```python
from build123d import *

# Parameters (mm, degrees)
SKETCH1_W           = 50.8
SKETCH1_H           = 25.4
SKETCH1_W_2         = 47.625
SKETCH1_H_2         = 22.225
BOSS_EXTRUDE1_DEPTH = 355.6
SKETCH2_R           = 12.7
SKETCH2_R_2         = 2.54
CUT_EXTRUDE4_DEPTH  = 32.766
CUT_EXTRUDE5_REACH  = 359.41


with BuildPart() as part:
    # Sketch1 → Boss-Extrude1 (new body)
    with BuildSketch(Plane.XY):
        Rectangle(SKETCH1_W, SKETCH1_H)
        Rectangle(SKETCH1_W_2, SKETCH1_H_2, mode=Mode.SUBTRACT)
    extrude(amount=BOSS_EXTRUDE1_DEPTH)

    # Sketch2 → Cut-Extrude4 (cut)
    with BuildSketch(Plane(origin=(0, 12.7, 0), x_dir=(1, 0, 0), z_dir=(0, 1, 0))):
        with Locations(Location((0, -177.8, 0), (0, 0, 180))):
            Circle(SKETCH2_R)
        with Locations(Location((0, -152.4, 0), (0, 0, 180))):
            Circle(SKETCH2_R_2)
        with Locations(Location((0, -201.676, 0), (0, 0, 180))):
            Circle(SKETCH2_R_2)
    extrude(amount=-CUT_EXTRUDE4_DEPTH, mode=Mode.SUBTRACT)

    # Sketch3 → Cut-Extrude5 (cut, up to next)
    with BuildSketch(Plane.XZ.offset(12.7), mode=Mode.PRIVATE) as cut_extrude5_sk1:
        with BuildLine():
            ThreePointArc((-4.48e-07, 355.6), (12.899331681, 354.46174048), (25.4, 351.082140551))
            Line((25.4, 351.082140551), (25.4, 355.6))
            Line((25.4, 355.6), (-4.48e-07, 355.6))
        make_face()
    cut_extrude5_tool1 = extrude(cut_extrude5_sk1.sketch, amount=-CUT_EXTRUDE5_REACH, mode=Mode.PRIVATE) & part.part
    # Sketch3 → Cut-Extrude5 (cut, up to next)
    with BuildSketch(Plane.XZ.offset(12.7), mode=Mode.PRIVATE) as cut_extrude5_sk2:
        with BuildLine():
            Line((-25.4, 355.6), (-25.4, 351.082140551))
            ThreePointArc((-25.4, 351.082140551), (-12.899332122, 354.461740401), (-4.48e-07, 355.6))
            Line((-4.48e-07, 355.6), (-25.4, 355.6))
        make_face()
    cut_extrude5_tool2 = extrude(cut_extrude5_sk2.sketch, amount=-CUT_EXTRUDE5_REACH, mode=Mode.PRIVATE) & part.part
    # Sketch3 → Cut-Extrude5 (cut, up to next)
    with BuildSketch(Plane.XZ.offset(12.7), mode=Mode.PRIVATE) as cut_extrude5_sk3:
        with BuildLine():
            ThreePointArc((25.4, 4.436419441), (12.892263223, 1.117437052), (-2.64e-07, 0))
            Line((-2.64e-07, 0), (25.4, 0))
            Line((25.4, 0), (25.4, 4.436419441))
        make_face()
    cut_extrude5_tool3 = extrude(cut_extrude5_sk3.sketch, amount=-CUT_EXTRUDE5_REACH, mode=Mode.PRIVATE) & part.part
    # Sketch3 → Cut-Extrude5 (cut, up to next)
    with BuildSketch(Plane.XZ.offset(12.7), mode=Mode.PRIVATE) as cut_extrude5_sk4:
        with BuildLine():
            Line((-25.4, 4.436419441), (-25.4, 0))
            Line((-25.4, 0), (-2.64e-07, 0))
            ThreePointArc((-2.64e-07, 0), (-12.892263483, 1.117437097), (-25.4, 4.436419441))
        make_face()
    cut_extrude5_tool4 = extrude(cut_extrude5_sk4.sketch, amount=-CUT_EXTRUDE5_REACH, mode=Mode.PRIVATE) & part.part
    add(cut_extrude5_tool1.solids().sort_by_distance((19.0896, -12.7, 354.252078))[0], mode=Mode.SUBTRACT)
    add(cut_extrude5_tool2.solids().sort_by_distance((-19.0896, -12.7, 354.252078))[0], mode=Mode.SUBTRACT)
    add(cut_extrude5_tool3.solids().sort_by_distance((19.088205, -12.7, 1.323888))[0], mode=Mode.SUBTRACT)
    add(cut_extrude5_tool4.solids().sort_by_distance((-19.088205, -12.7, 1.323888))[0], mode=Mode.SUBTRACT)


solid = part.part
```
For this review, take the finished solid that the model builds, in its own axes (mm). A direction names the side the tool comes from. Coordinates: 2 decimals unless noted, no trailing zeros. Order: outer loops, then holes, each group sorted by start corner. A loop starts at its lowest first (then second) coordinate and runs counter-clockwise, first axis right, second up. Notation, with made-up numbers: (37, -12.5) - (64, -12.5) arc R31 cw to (64, 25.5) - close; hole circle Ø3 at (14, 50). An arc over 180 degrees is marked (long way). Answer as a JSON object with one key per item and string values. Group by question number.
1. Clearance check with flat-ended pins moving along their axes: P1, Ø20.5, axis at x = 0, z = 177.8, coming from the -Y side (1 decimal); P2, Ø8, axis at x = -7.5, y = -8, coming from the -Z side; P3, Ø6, axis at x = 0, z = 152.4, coming from the +Y side. State where each tip first meets the part, or that it passes through.
2. We need section B-B on y = -5.75. State the section outline as (x, z) points.
3. For probe 1 along Z at (x, y) = (0, -11.75); probe 2 along Y at (x, z) = (9, 106); probe 3 along X at (y, z) = (12.35, 152.4), list the stretches that pass through material, from the lowest coordinate up.
4. The part is to be moulded in two halves that separate along X. For faces 3 (the flat face through (17, -12.7, 175)), 4 (the flat face through (-16, -11.112, 175)), 5 (the flat face through (-25.4, 0, 175)), 6 (the flat face through (25.4, 0, 175)), say which applies: pulls with the +X half, pulls with the -X half, needs draft (parallel to the pull), parting line crosses it, or undercut.
5. We need section A-A on z = 138. State the section outline as (x, y) points.
6. We need section C-C on z = 177.8. State the section outline as (x, y) points.
7. For faces 1 (the flat face through (-23.812, 0, 175)), 2 (the flat face through (17, 12.7, 175)), list the 3-axis set-ups (+Z, -Z, +X, -X, +Y, -Y) from which the entire face can be reached by the end or side of a thin tool; tool diameter is ignored.
Final values:
{
 "1": {"P1": "through", "P2": "z = 0.17", "P3": "y = 12.7"},
 "2": {"outline": "(-25.4, 4.44) arc R74.93 ccw to (-23.81, 3.88) - (-23.81, 351.64) arc R73.66 ccw to (-25.4, 351.08) - close; (23.81, 3.88) arc R74.93 ccw to (25.4, 4.44) - (25.4, 351.08) arc R73.66 ccw to (23.81, 351.64) - close"},
 "3": {"probe 1": "0 to 149.86, 154.94 to 165.1, 190.5 to 199.14, 204.22 to 355.6", "probe 2": "-12.7 to -11.11, 11.11 to 12.7", "probe 3": "-25.4 to -2.54, 2.54 to 25.4"},
 "4": {"face 3": "needs draft", "face 4": "undercut", "face 5": "pulls with the -X half", "face 6": "pulls with the +X half"},
 "5": {"outline": "(-25.4, -12.7) - (25.4, -12.7) - (25.4, 12.7) - (-25.4, 12.7) - close; hole (-23.81, -11.11) - (23.81, -11.11) - (23.81, 11.11) - (-23.81, 11.11) - close"},
 "6": {"outline": "(-25.4, -12.7) - (-12.7, -12.7) - (-12.7, -11.11) - (-23.81, -11.11) - (-23.81, 11.11) - (-12.7, 11.11) - (-12.7, 12.7) - (-25.4, 12.7) - close; (12.7, -12.7) - (25.4, -12.7) - (25.4, 12.7) - (12.7, 12.7) - (12.7, 11.11) - (23.81, 11.11) - (23.81, -11.11) - (12.7, -11.11) - close"},
 "7": {"face 1": "+Z, -Z", "face 2": "+Z, -Z, +X, -X, +Y"}
}
